Autodesk Inventor part; units mm, degrees
ref_plane "YZ Plane" through (0, 0, 0) normal (1, 0, 0) x (0, 1, 0)
ref_plane "XZ Plane" through (0, 0, 0) normal (0, 1, 0) x (-1, 0, 0)
ref_plane "XY Plane" through (0, 0, 0) normal (0, 0, 1) x (1, 0, 0)
sketch "Sketch1" plane through (0, 0, 0) normal (0, 0, 1) x (1, 0, 0)
  line L0 (-50, -53.5) -> (50, -53.5)
  line L1 (50, -53.5) -> (50, 53.5)
  line L2 (50, 53.5) -> (-50, 53.5)
  line L3 (-50, 53.5) -> (-50, -53.5)
  line L4 (-50, -53.5) -> (50, 53.5) construction
  line L5 (50, -53.5) -> (-50, 53.5) construction
  point P0 (0, 0)
  dimension "d154" = 100
  dimension "d155" = 107
extrude "Plate5" add sketch "Sketch1" along normal blind 3
sketch "Sketch9" plane through (0, 0, 0) normal (0, 0, -1) x (-1, 0, 0)
  line L0 (25.75, -33.25) -> (-9.75, -33.25)
  line L1 (-9.75, -33.25) -> (-9.75, 2.25)
  line L2 (-9.75, 2.25) -> (25.75, 2.25)
  line L3 (25.75, 2.25) -> (25.75, -33.25)
  line L4 (25.75, -33.25) -> (-9.75, 2.25) construction
  line L5 (-9.75, -33.25) -> (25.75, 2.25) construction
  circle A0 centre (34.5165, -42.0165) radius 2.5
  circle A1 centre (-18.5165, -42.0165) radius 2.5
  circle A2 centre (-18.5165, 11.0165) radius 2.5
  circle A3 centre (34.5165, 11.0165) radius 2.5
  circle A4 centre (8, -15.5) radius 37.5 construction
  line L6 (-9.75, -33.25) -> (-18.5165, -42.0165) construction
  line L7 (50, 53.5) -> (50, -53.5)
  line L8 (-50, -53.5) -> (-50, 53.5)
  line L9 (50, -53.5) -> (-50, -53.5)
  line L10 (50, 53.5) -> (50, -53.5)
  line L11 (-50, 53.5) -> (50, 53.5)
  point P0 (0, 0)
  dimension "d173" = 35.5
  dimension "d174" = 35.5
  dimension "d175" = 5
  dimension "d176" = 12.3977
  dimension "d179" = 42
  dimension "d180" = 69
  dimension "d183" = 75
extrude "Extrusion3" cut sketch "Sketch9" against normal blind 10 contours L0 L1 L2 L3 | A0 | A1 | A2 | A3
sketch "Sketch7" plane through (-47, -53.5, 0) normal (-1, 0, 0) x (0, -1, 0)
  line L0 (-107, 0) -> (0, 0)
  line L1 (0, 0) -> (0, 84)
  line L2 (0, 84) -> (-107, 84)
  line L3 (-107, 84) -> (-107, 0)
edge flange "Flange3" height 84 angle 90 thickness 3 bend radius 2.75 thickness toward (-1, 0, 0) relief round relief width 3 relief depth 1.5 edges at (-50, 0, 3) wall of the first edge with corners at (-47, 53.5, 0) (-47, -53.5, 0) (-47, -53.5, 84) (-47, 53.5, 84)
bend "Bend3"
corner "Corner3"
properties part number "PNS 753 FDS 1200 FLANGE 2 up" material "Stainless Steel"
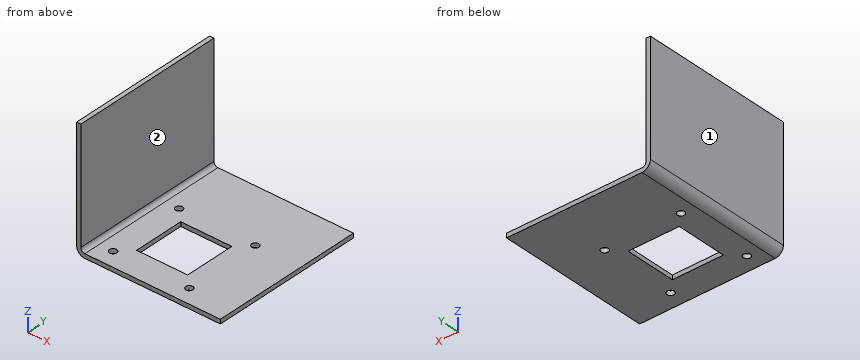
Can you work these out from the model? Positions are in its coordinate system, mm. Face numbers are marked on the shaded views. A direction names the side the tool comes from. Coordinates: 2 decimals unless noted, no trailing zeros. Loops run counter-clockwise (first coordinate to the right, second up) from the corner with the lowest first, then second, coordinate; pieces in that order, holes last. Notation, with made-up numbers: (-16.5, -1) -> (34.5, -1) arc R19 cw to (34.5, 16) -> close; hole circle Ø2 at (62.5, 13.25). An arc over 180 degrees is marked (long way). Answer as a JSON object with one key per item and string values.
1) For P1, Ø5, axis at x = 15, y = -31.5, coming from the +Z side; P2, Ø0.9, axis at y = -18.5, z = 2, coming from the -X side; P3, Ø2, axis at y = 0, z = 57.5, coming from the +X side; P4, Ø6, axis at x = -34.52, y = 11.02, coming from the -Z side, each with a flat end and sliding along its axis, tell me the tip position at first contact or that it passes through.
Results:
{"P1": "stops at z = 3", "P2": "stops at x = -48.96", "P3": "stops at x = -47", "P4": "stops at z = 0"}
2) For the marked faces 1 and 2, which set-ups out of +Z, -Z, +X, -X, +Y, -Y let a thin tool reach every point of the face, with its end or its side?
Results:
{"face 1": "+Z, -Z, -X, +Y, -Y", "face 2": "+Z, +X, +Y, -Y"}
3) If I drill on line 1 (X direction, y = 31, z = 45); line 2 (Z direction, x = 1, y = 15.5), over which ranges is the centre line in solid material (lowest first)?
Results:
{"line 1": "x = -50 to -47", "line 2": "z = 0 to 3"}
4) Imagine slicing it at D-D (z = 30). Please give me the cut outline in (x, y), then the cut area to 3 significant figures.
Results:
{"outline": "(-50, -53.5) -> (-47, -53.5) -> (-47, 53.5) -> (-50, 53.5) -> close", "area": "321 mm^2"}
5) Imagine slicing it at B-B (y = 34.5). Please give me the cut outline in (x, z).
Results:
{"outline": "(-50, 5.75) arc R5.75 ccw to (-44.25, 0) -> (50, 0) -> (50, 3) -> (-44.25, 3) arc R2.75 cw to (-47, 5.75) -> (-47, 84) -> (-50, 84) -> close"}
6) Imagine slicing it at C-C (x = 26). Please give me the cut outline in (y, z).
Results:
{"outline": "(-53.5, 0) -> (53.5, 0) -> (53.5, 3) -> (-53.5, 3) -> close"}
7) Imagine slicing it at A-A (y = -23). Please give me the cut outline in (x, z), then the cut area to 3 significant figures.
Results:
{"outline": "(-50, 5.75) arc R5.75 ccw to (-44.25, 0) -> (-25.75, 0) -> (-25.75, 3) -> (-44.25, 3) arc R2.75 cw to (-47, 5.75) -> (-47, 84) -> (-50, 84) -> close; (9.75, 0) -> (50, 0) -> (50, 3) -> (9.75, 3) -> close", "area": "431 mm^2"}
